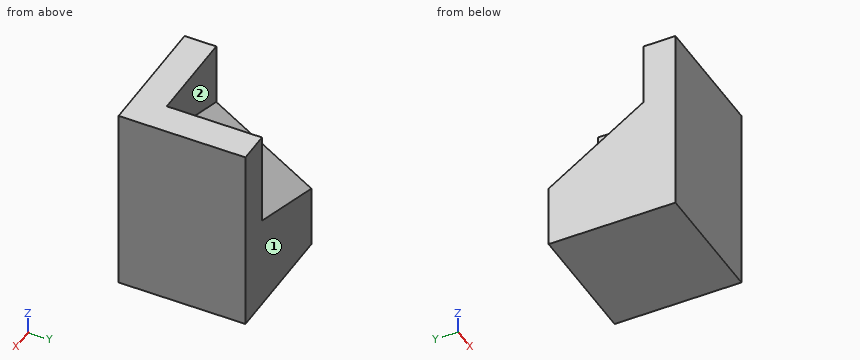
from build123d import *

# Parameters (mm, degrees)
SKETCH_10_W         = 60
SKETCH_10_H         = 40
EXTRUDE_3_DEPTH     = 40
CUT_EXTRUDE_2_DEPTH = 30


with BuildPart() as part:
    # 草圖10 → 填料-伸長3 (new body)
    with BuildSketch(Plane(origin=(0, 0, 0), x_dir=(0, 0, -1), z_dir=(1, 0, 0))):
        with Locations((-2.876712329, 15.643835616)):
            Rectangle(SKETCH_10_W, SKETCH_10_H)
    extrude(amount=EXTRUDE_3_DEPTH)

    # 草圖11 → 除料-伸長2 (cut)
    with BuildSketch(Plane(origin=(0, 35.643835616, 0), x_dir=(1, 0, 0), z_dir=(0, 1, 0))):
        Polygon((0, -12.876712329), (30, -22.876712329), (30, -32.876712329), (0, -32.876712329), align=None)
    extrude(amount=-CUT_EXTRUDE_2_DEPTH, mode=Mode.SUBTRACT)

    # 除料-掃出1: sweep along a path in 草圖13
    with BuildLine(Plane(origin=(0, 5.643835616, 0), x_dir=(1, 0, 0), z_dir=(0, 1, 0))) as sweep_1_path:
        Line((30, -22.876712329), (0, -12.876712329))
    # 草圖12 → 除料-掃出1 (sweep, cut)
    with BuildSketch(Plane.ZY.offset(-30)):
        Polygon((22.876712329, 5.643835616), (2.876712329, 35.643835616), (32.876712329, 35.643835616), (32.876712329, 5.643835616), align=None)
    sweep(path=sweep_1_path.line, mode=Mode.SUBTRACT)


solid = part.part
Build history of the part. All positions in model axes, mm. Face numbers are marked on the shaded views. A direction names the side the tool comes from. Give positions to 0.01 mm unless a question says otherwise; leave off trailing zeros. Write each loop counter-clockwise with the first axis right and the second up, starting at its lowest first coordinate (ties: lowest second). Pieces come first, ordered by that corner, then holes. Notation, with made-up numbers: (63, -3) - (104, -3) arc R31 ccw to (104, 36) - close; hole circle Ø4 at (81, 4). An arc over 180 degrees is marked (long way). Use one line per item in the form item = value. Start each with the question number.
1. 3-axis set-ups, long thin cutter, end or side, ignore diameter. For the marked faces 1 and 2: which of +Z, -Z, +X, -X, +Y, -Y reach the whole face in a straight line?
2. Band-saw the part on C-C on z = 18. Write the cut outline in (x, y), plus the area to 3 significant figures.
3. Band-saw the part on D-D on z = -2. Write the cut outline in (x, y).
4. Drop flat-ended pins along their axis: pin 1 Ø5 at (x, y) = (20, 17.5) entering from +Z; pin 2 Ø12 at (x, y) = (5, 18.5) entering from +Z; pin 3 Ø10 at (x, z) = (10, 18) entering from +Y. Give the stop position or say it passes through.
5. Band-saw the part on B-B on x = 3. Write the cut outline in (y, z), plus the area to 3 significant figures.
6. Band-saw the part on A-A on z = 29. Write the cut outline in (x, y).
7. Probe line 1 (Y direction, x = 17, z = 19); line 2 (X direction, y = 11.5, z = 23.5); line 3 (Z direction, x = 29, y = 6.5). List the from-to ranges inside material, lowest first. Write a range as [from, to].
Conclusion:
q1.face_1 = +Z, -Z, +X, -X, +Y
q1.face_2 = +Z, -X, +Y
q2.outline = (0, -4.36) - (40, -4.36) - (40, 35.64) - (30, 35.64) - (30, 12.96) - (15.37, 5.64) - (0, 5.64) - close
q2.area = 754 mm²
q3.outline = (0, -4.36) - (40, -4.36) - (40, 35.64) - (15.37, 35.64) - (0, 27.96) - close
q4.pin_1 = 13.5
q4.pin_2 = 10.44
q4.pin_3 = 10.86
q5.outline = (-4.36, -27.12) - (35.64, -27.12) - (35.64, -6.12) - (5.64, 13.88) - (5.64, 32.88) - (-4.36, 32.88) - close
q5.area = 1,530 mm²
q6.outline = (0, -4.36) - (40, -4.36) - (40, 35.64) - (30, 35.64) - (30, 5.64) - (0, 5.64) - close
q7.line_1 = [-4.36, 5.64]
q7.line_2 = [30, 40]
q7.line_3 = [-27.12, 21.97]
